```python
from build123d import *

# Parameters (mm, degrees)
SKETCH1_W           = 8.5
SKETCH1_H           = 8.5
BOSS_EXTRUDE1_DEPTH = 5
SKETCH2_W           = 8.5
SKETCH2_H           = 8.5
BOSS_EXTRUDE2_DEPTH = 2
SKETCH3_R           = 1.5
CUT_EXTRUDE1_DEPTH  = 2
SKETCH4_W           = 53.5
SKETCH4_H           = 8.5
BOSS_EXTRUDE3_DEPTH = 3
SKETCH5_W           = 7
SKETCH5_H           = 8.5
BOSS_EXTRUDE4_DEPTH = 8.5
SKETCH8_R           = 1.5
BOSS_EXTRUDE5_DEPTH = 2.5
SKETCH10_W          = 8.5
SKETCH10_H          = 8.5
BOSS_EXTRUDE7_DEPTH = 1
CUT_EXTRUDE4_DEPTH  = 0.5
SKETCH14_W          = 8.5
SKETCH14_H          = 8.5
BOSS_EXTRUDE8_DEPTH = 8
SKETCH15_W          = 8.5
SKETCH15_H          = 8.5
CUT_EXTRUDE6_DEPTH  = 1
SKETCH16_W          = 53.5
SKETCH16_H          = 3.5
CUT_EXTRUDE7_DEPTH  = 15
SKETCH17_W          = 5
SKETCH17_H          = 8.5
BOSS_EXTRUDE9_DEPTH = 7


with BuildPart() as part:
    # Sketch1 → Boss-Extrude1 (new body)
    with BuildSketch(Plane(origin=(0, 0, 0), x_dir=(0, 0, -1), z_dir=(1, 0, 0))):
        Rectangle(SKETCH1_W, SKETCH1_H)
        Polygon((1.705, 2.953146627), (-1.705, 2.953146627), (-3.41, 0), (-1.705, -2.953146627), (1.705, -2.953146627), (3.41, 0), align=None, mode=Mode.SUBTRACT)
    extrude(amount=BOSS_EXTRUDE1_DEPTH)

    # Sketch2 → Boss-Extrude2 (add)
    with BuildSketch(Plane.ZY):
        Rectangle(SKETCH2_W, SKETCH2_H)
    extrude(amount=BOSS_EXTRUDE2_DEPTH)

    # Sketch3 → Cut-Extrude1 (cut)
    with BuildSketch(Plane(origin=(0, 0, 0), x_dir=(0, 0, -1), z_dir=(1, 0, 0))):
        Circle(SKETCH3_R)
    extrude(amount=-CUT_EXTRUDE1_DEPTH, mode=Mode.SUBTRACT)

    # Sketch4 → Boss-Extrude3 (add)
    with BuildSketch(Plane.XZ.offset(4.25)):
        with Locations((24.75, 0)):
            Rectangle(SKETCH4_W, SKETCH4_H)
    extrude(amount=BOSS_EXTRUDE3_DEPTH)

    # Sketch5 → Boss-Extrude4 (add)
    with BuildSketch(Plane(origin=(0, -4.25, 0), x_dir=(1, 0, 0), z_dir=(0, 1, 0))):
        with Locations((48, 0)):
            Rectangle(SKETCH5_W, SKETCH5_H)
    extrude(amount=BOSS_EXTRUDE4_DEPTH)

    # Sketch8 → Boss-Extrude5 (add)
    with BuildSketch(Plane(origin=(0, 0, 0), x_dir=(0, 0, -1), z_dir=(1, 0, 0))):
        Polygon((-1.705, 2.953146627), (-3.41, 0), (-1.705, -2.953146627), (1.705, -2.953146627), (3.41, 0), (1.705, 2.953146627), align=None)
        Circle(SKETCH8_R, mode=Mode.SUBTRACT)
    extrude(amount=BOSS_EXTRUDE5_DEPTH)

    # Sketch10 → Boss-Extrude7 (add)
    with BuildSketch(Plane(origin=(5, 0, 0), x_dir=(0, 0, -1), z_dir=(1, 0, 0))):
        Rectangle(SKETCH10_W, SKETCH10_H)
        Polygon((3.41, 0), (1.705, 2.953146627), (-1.705, 2.953146627), (-3.41, 0), (-1.705, -2.953146627), (1.705, -2.953146627), align=None, mode=Mode.SUBTRACT)
    extrude(amount=BOSS_EXTRUDE7_DEPTH)

    # Sketch12 → Cut-Extrude4 (cut)
    with BuildSketch(Plane(origin=(2.5, 0, 0), x_dir=(0, 0, -1), z_dir=(1, 0, 0))):
        Polygon((1.705, -2.953146627), (3.41, 0), (1.705, 2.953146627), (-1.705, 2.953146627), (-3.41, 0), (-1.705, -2.953146627), align=None)
    extrude(amount=-CUT_EXTRUDE4_DEPTH, mode=Mode.SUBTRACT)

    # Sketch14 → Boss-Extrude8 (add)
    with BuildSketch(Plane(origin=(6, 0, 0), x_dir=(0, 0, -1), z_dir=(1, 0, 0))):
        Rectangle(SKETCH14_W, SKETCH14_H)
    extrude(amount=-BOSS_EXTRUDE8_DEPTH)

    # Sketch15 → Cut-Extrude6 (cut)
    with BuildSketch(Plane(origin=(6, 0, 0), x_dir=(0, 0, -1), z_dir=(1, 0, 0))):
        Rectangle(SKETCH15_W, SKETCH15_H)
    extrude(amount=-CUT_EXTRUDE6_DEPTH, mode=Mode.SUBTRACT)

    # Sketch16 → Cut-Extrude7 (cut)
    with BuildSketch(Plane(origin=(0, 4.25, 0), x_dir=(1, 0, 0), z_dir=(0, 1, 0))):
        with Locations((24.75, 2.5)):
            Rectangle(SKETCH16_W, SKETCH16_H)
    extrude(amount=-CUT_EXTRUDE7_DEPTH, mode=Mode.SUBTRACT)

    # Sketch17 → Boss-Extrude9 (add)
    with BuildSketch(Plane.ZY.offset(-44.5)):
        with Locations((1.75, 0)):
            Rectangle(SKETCH17_W, SKETCH17_H)
    extrude(amount=-BOSS_EXTRUDE9_DEPTH)


solid = part.part
```
Design review of the part built by this model. Coordinates are the model's own, in mm. A direction names the side the tool comes from. Round coordinates to 2 decimals unless told otherwise and drop trailing zeros. Write each loop counter-clockwise with the first axis right and the second up, starting at its lowest first coordinate (ties: lowest second). Pieces come first, ordered by that corner, then holes. Notation, with made-up numbers: (-38.75, 78) -> (-0.75, 78) arc R18 cw to (-0.75, 112) -> close; hole circle Ø2 at (-8.5, -7). An arc over 180 degrees is marked (long way). Write item = value, one per line. Start each with the question number.
1) Take a section at B-B, the plane z = 2.65. State the section outline as (x, y) points, plus the area to 4 significant figures.
2) Mouldability with a two-part tool opening along X and no side actions: class faces 3 (the face through (48, 4.25, 2)), 4 (the face through (24, -4.25, 2)), 5 (the face through (-2, -1, 2)), 6 (the face through (51.5, -2, 2)) as +X half, -X half, draft (parallel to the pull), parting line (faces both ways), or undercut.
3) Wall thickness on probe 1 along X at (y, z) = (-1.75, 0); probe 2 along Y at (x, z) = (22.5, 0.15): over which ranges is each line inside the solid? List them lowest first. Write a range as from..to.
4) Tool access review of faces 1 (the face through (1, 4.25, 2)), 2 (the face through (5, 0, 2)): name each direction out of +Z, -Z, +X, -X, +Y, -Y from which nothing blocks a thin tool from reaching the whole face with its end or side.
5) Clearance check with a flat-ended pin moving along its axis: pin 1 (2 mm diameter, centred on x = 38.5, z = 0.5, fed in from +Y). State where the tip first meets the part, or that it passes through.
6) Take a section at C-C, the plane x = 27. State the section outline as (y, z) points.
7) Take a section at A-A, the plane y = -2.5. State the section outline as (x, z) points.
Results list:
q1.outline = (-2, -7.25) -> (51.5, -7.25) -> (51.5, 4.25) -> (44.5, 4.25) -> (44.5, -4.25) -> (5, -4.25) -> (5, 4.25) -> (-2, 4.25) -> close
q1.area = 279.5 mm²
q2.face_3 = draft
q2.face_4 = undercut
q2.face_5 = -X half
q2.face_6 = +X half
q3.probe_1 = -2..5, 44.5..51.5
q3.probe_2 = -7.25..-4.25
q4.face_1 = +Z, -Z, +X, -X, +Y
q4.face_2 = +Z, -Z, +Y
q5.pin_1 = -4.25
q6.outline = (-7.25, -0.75) -> (-4.25, -0.75) -> (-4.25, 4.25) -> (-7.25, 4.25) -> close
q7.outline = (-2, -0.75) -> (5, -0.75) -> (5, 4.25) -> (-2, 4.25) -> close; (44.5, -0.75) -> (51.5, -0.75) -> (51.5, 4.25) -> (44.5, 4.25) -> close
